Build history of the part. All positions in model axes, mm. Face numbers are marked on the shaded views. A direction names the side the tool comes from. Coordinates: 2 decimals unless noted, no trailing zeros. Write each loop counter-clockwise with the first axis right and the second up, starting at its lowest first coordinate (ties: lowest second). Pieces come first, ordered by that corner, then holes.
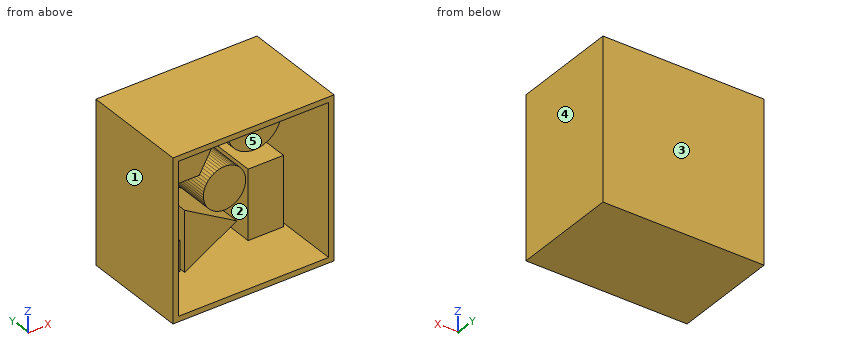
```python
from build123d import *

# Parameters (mm, degrees)
F0_W      = 74.9482437968
F0_H      = 75.0057548285
F1_DEPTH  = 25
F2_DEPTH  = 25
F3_T      = -2.5
F5_DEPTH  = 25
F6_R      = 12.6957463679
F7_DEPTH  = 25
F8_W      = 16.4368115366
F8_H      = 32.2714154609
F9_DEPTH  = 25
F11_DEPTH = 25
F12_W     = 13.7684866786
F12_H     = 13.7785351835
F13_DEPTH = 25
F15_DEPTH = 25


with BuildPart() as f1:
    # F0 (on Front) → F1 (new body)
    with BuildSketch(Plane.XZ):
        with Locations((-37.4741218984, 37.5028774142)):
            Rectangle(F0_W, F0_H)
    extrude(amount=F1_DEPTH)

    # F2 (add): a face of the model
    f2_faces = [f1.faces().sort_by_distance(p)[0] for p in [
        (-37.4741218984, 0, 37.5028774142),
    ]]
    extrude(f2_faces, amount=F2_DEPTH)

    # F3
    f3_openings = [f1.faces().sort_by_distance(p)[0] for p in [
        (-37.474122, -25, 37.502877),
    ]]
    offset(amount=F3_T, openings=f3_openings)

    # F4 (on face) → F5 (join)
    with BuildSketch(Plane.XZ.offset(-22.5)):
        Polygon((-46.5854653187, 44.4409851923), (-38.8256809644, 58.027296792), (-46.7118797764, 71.5406229706), (-62.3578629427, 71.4676375494), (-70.1176472969, 57.8813259497), (-62.231448485, 44.3679997711), align=None)
    extrude(amount=F5_DEPTH)

    # F6 (on face) → F7 (join)
    with BuildSketch(Plane.XZ.offset(-22.5)):
        with Locations((-20.9236498922, 58.88639763)):
            Circle(F6_R)
    extrude(amount=F7_DEPTH)

    # F8 (on face) → F9 (join)
    with BuildSketch(Plane.XZ.offset(-22.5)):
        with Locations((-15.6277697533, 22.4080828484)):
            Rectangle(F8_W, F8_H)
    extrude(amount=F9_DEPTH)

    # F10 (on face) → F11 (join)
    with BuildSketch(Plane.XZ.offset(-22.5)):
        Polygon((-53.3962547779, 31.2044414208), (-53.3962547779, 3.1478276029), (-29.0985144675, 17.1761345118), align=None)
    extrude(amount=F11_DEPTH)

    # F12 (on face) → F13 (join)
    with BuildSketch(Plane.XZ.offset(-22.5)):
        with Locations((-62.4265633523, 11.3765813876)):
            Rectangle(F12_W, F12_H)
    extrude(amount=F13_DEPTH)

    # F14 (on face) → F15 (join)
    with BuildSketch(Plane.XZ.offset(-22.5)):
        Polygon((-44.6300245821, 34.7623496997), (-44.6300245821, 33.5300371302), (-44.475574863, 32.3074417133), (-44.1691111892, 31.1138445092), (-43.7154666758, 29.9680692588), (-43.1217955677, 28.8881855222), (-42.3974604132, 27.8912237111), (-41.5538844101, 26.9929065087), (-40.604371256, 26.207400914), (-39.5638953406, 25.5470948195), (-38.4488655906, 25.0224016466), (-37.2768666912, 24.6415961203), (-36.0663817653, 24.410683771), (-34.8365008831, 24.3333062246), (-33.6066200009, 24.410683771), (-32.396135075, 24.6415961203), (-31.2241361756, 25.0224016466), (-30.1091064256, 25.5470948195), (-29.0686305102, 26.207400914), (-28.1191173561, 26.9929065087), (-27.2755413531, 27.8912237111), (-26.5512061985, 28.8881855222), (-25.9575350905, 29.9680692588), (-25.503890577, 31.1138445092), (-25.1974269032, 32.3074417133), (-25.0429771841, 33.5300371302), (-25.0429771841, 34.7623496997), (-25.1974269032, 35.9849451165), (-25.503890577, 37.1785423206), (-25.9575350905, 38.3243175711), (-26.5512061985, 39.4042013076), (-27.2755413531, 40.4011631188), (-28.1191173561, 41.2994803211), (-29.0686305102, 42.0849859158), (-30.1091064256, 42.7452920104), (-31.2241361756, 43.2699851832), (-32.396135075, 43.6507907096), (-33.6066200009, 43.8817030588), (-34.8365008831, 43.9590806053), (-36.0663817653, 43.8817030588), (-37.2768666912, 43.6507907096), (-38.4488655906, 43.2699851832), (-39.5638953406, 42.7452920104), (-40.604371256, 42.0849859158), (-41.5538844101, 41.2994803211), (-42.3974604132, 40.4011631188), (-43.1217955677, 39.4042013076), (-43.7154666758, 38.3243175711), (-44.1691111892, 37.1785423206), (-44.475574863, 35.9849451165), align=None)
    extrude(amount=F15_DEPTH)


solid = f1.part
```
1. 3-axis set-ups, long thin cutter, end or side, ignore diameter. For the marked faces 1 and 2: which of +Z, -Z, +X, -X, +Y, -Y reach the whole face in a straight line?
Computed values:
face 1: +Z, -Z, -X, +Y, -Y
face 2: -Y
2. Flat gauge pins, fed straight in: pin 1 (4 mm diameter, centred on y = -17.5, z = 42, fed in from +X); pin 2 (5 mm diameter, centred on x = -18, z = 22.5, fed in from -Y). Where does each tip first touch, or does it go through?
Computed values:
pin 1: stops at x = 0
pin 2: stops at y = -2.5
3. Mould opens along X. For the marked faces 3, 4 and 5 say: +X half, -X half, draft (parallel to the pull), parting line (faces both ways), or undercut.
Computed values:
face 3: draft
face 4: +X half
face 5: undercut
4. Saw through at D-D on y = 4. State how many separate pieces and enclosed holes the cut face has, plus the area to 3 significant figures.
Computed values:
separate pieces: 7
enclosed holes: 1
area: 3,230 mm2
5. Probe line 1 along Z through (x, y) = (-61, 1); line 2 along X through (y, z) = (-12.5, 32); line 3 along Z through (x, y) = (-9, -11.5). List the from-to ranges inside material, lowest first.
Computed values:
line 1: z = 0 to 2.5, 4.49 to 18.27, 44.37 to 71.47, 72.51 to 75.01
line 2: x = -74.95 to -72.45, -2.5 to 0
line 3: z = 0 to 2.5, 72.51 to 75.01
6. Saw through at C-C on x = -57. List the corners of the cut face in (y, z), plus the area to 3 significant figures.
Computed values:
outline: (-25, 0) - (25, 0) - (25, 75.01) - (-25, 75.01) - (-25, 72.51) - (22.5, 72.51) - (22.5, 71.49) - (-2.5, 71.49) - (-2.5, 44.39) - (22.5, 44.39) - (22.5, 18.27) - (-2.5, 18.27) - (-2.5, 4.49) - (22.5, 4.49) - (22.5, 2.5) - (-25, 2.5) - close
area: 1,450 mm2
7. Saw through at A-A on y = -20.5. List the corners of the cut face in (x, z).
Computed values:
outline: (-74.95, 0) - (0, 0) - (0, 75.01) - (-74.95, 75.01) - close; hole (-72.45, 2.5) - (-2.5, 2.5) - (-2.5, 72.51) - (-72.45, 72.51) - close
8. Saw through at B-B on z = 62. List the corners of the cut face in (x, y).
Computed values:
outline: (-74.95, -25) - (-72.45, -25) - (-72.45, 22.5) - (-67.77, 22.5) - (-67.77, -2.5) - (-41.14, -2.5) - (-41.14, 22.5) - (-33.23, 22.5) - (-33.23, -2.5) - (-8.62, -2.5) - (-8.62, 22.5) - (-2.5, 22.5) - (-2.5, -25) - (0, -25) - (0, 25) - (-74.95, 25) - close
